Geometry check sheet. Reference: the model listing, model coordinates, mm. A direction names the side the tool comes from. Give positions to 0.01 mm unless a question says otherwise; leave off trailing zeros. Order: outer loops, then holes, each group sorted by start corner. A loop starts at its lowest first (then second) coordinate and runs counter-clockwise, first axis right, second up. Notation, with made-up numbers: M 1,-19.5 L 45,-19.5 A24 cw 45,-5.5 Z; hole C -17.75,-11.75 d9. An arc over 180 degrees is marked long. Answer as CSV lines item,"result".
from build123d import *

# Parameters (mm, degrees)
SKETCH1_R           = 2.625
BOSS_EXTRUDE1_DEPTH = 3.175


with BuildPart() as part:
    # Sketch1 → Boss-Extrude1 (new body)
    with BuildSketch(Plane.XY):
        Polygon((-8.910000095, 8.69), (6.789999905, 8.69), (6.789999905, 60.853549492), (88.409998474, 60.853549492), (88.409998474, 8.69), (104.109998474, 8.69), (104.109998474, 75.81), (88.409998474, 75.81), (6.789999905, 75.81), (-8.910000095, 75.81), align=None)
        with Locations((-2.560000095, 53.76)):
            Circle(SKETCH1_R, mode=Mode.SUBTRACT)
        with Locations((-2.560000095, 15.04)):
            Circle(SKETCH1_R, mode=Mode.SUBTRACT)
        with Locations((97.759998474, 15.04)):
            Circle(SKETCH1_R, mode=Mode.SUBTRACT)
        with Locations((97.759998474, 53.76)):
            Circle(SKETCH1_R, mode=Mode.SUBTRACT)
    extrude(amount=BOSS_EXTRUDE1_DEPTH)


solid = part.part
(1) Section check D-D on y = 15.04. Enter the section's corners in (x, z) (3 decimals).
The answers:
outline,"M -8.91,0 L -5.185,0 L -5.185,3.175 L -8.91,3.175 Z; M 0.065,0 L 6.79,0 L 6.79,3.175 L 0.065,3.175 Z; M 88.41,0 L 95.135,0 L 95.135,3.175 L 88.41,3.175 Z; M 100.385,0 L 104.11,0 L 104.11,3.175 L 100.385,3.175 Z"
(2) Material ranges on line 1 (Y direction, x = -2.56, z = 2.35) (3 decimals); line 2 (X direction, y = 15, z = 2.75); line 3 (X direction, y = 19.5, z = 2.45), recorded low to high.
The answers:
line 1,"y = 8.69 to 12.415, 17.665 to 51.135, 56.385 to 75.81"
line 2,"x = -8.91 to -5.18, 0.06 to 6.79, 88.41 to 95.14, 100.38 to 104.11"
line 3,"x = -8.91 to 6.79, 88.41 to 104.11"
(3) Tool access check on faces 1 (the face through (-8.91, 43, 2)), 2 (the face through (88.41, 35, 2)). Record the directions out of +Z, -Z, +X, -X, +Y, -Y that give a thin tool (end or side, any length) a straight path to the whole face; none if there is none.
The answers:
face 1,"+Z, -Z, -X, +Y, -Y"
face 2,"+Z, -Z, -Y"
(4) Section check A-A on x = -2.56. Enter the section's corners in (y, z) (3 decimals), then the cut area to 3 significant figures.
The answers:
outline,"M 8.69,0 L 12.415,0 L 12.415,3.175 L 8.69,3.175 Z; M 17.665,0 L 51.135,0 L 51.135,3.175 L 17.665,3.175 Z; M 56.385,0 L 75.81,0 L 75.81,3.175 L 56.385,3.175 Z"
area,"180 mm2"
(5) Section check B-B on y = 41.5. Enter the section's corners in (x, z) (3 decimals).
The answers:
outline,"M -8.91,0 L 6.79,0 L 6.79,3.175 L -8.91,3.175 Z; M 88.41,0 L 104.11,0 L 104.11,3.175 L 88.41,3.175 Z"
(6) Section check C-C on z = 2.3. Enter the section's corners in (x, y) (3 decimals).
The answers:
outline,"M -8.91,8.69 L 6.79,8.69 L 6.79,60.854 L 88.41,60.854 L 88.41,8.69 L 104.11,8.69 L 104.11,75.81 L -8.91,75.81 Z; hole C -2.56,15.04 d5.25; hole C -2.56,53.76 d5.25; hole C 97.76,15.04 d5.25; hole C 97.76,53.76 d5.25"
(7) Draft check along Y on faces 3 (the face through (47, 60.854, 2)), 4 (the face through (100.185, 52.755, 1.565)), 5 (the face through (6.79, 34, 2)). Enter one of: +Y half, -Y half, draft (parallel to the pull), parting line (faces both ways), or undercut.
The answers:
face 3,"-Y half"
face 4,"undercut"
face 5,"draft"
(8) Gauge pin test, flat ends, axial feed: P1, Ø1.5, axis at x = 32, z = 2, coming from the -Y side; P2, Ø4.5, axis at x = -2.56, y = 15.04, coming from the +Z side. Record the tip position at first contact, or that the pin passes through.
The answers:
P1,"stops at y = 60.85"
P2,"passes through"
